For this review, take the finished solid that the model builds, in its own axes (mm). A direction names the side the tool comes from. Coordinates: 2 decimals unless noted, no trailing zeros. Write each loop counter-clockwise with the first axis right and the second up, starting at its lowest first coordinate (ties: lowest second). Pieces come first, ordered by that corner, then holes. Notation, with made-up numbers: M 50,-37 L 76,-37 A17 ccw 76,-33 Z; hole C -33.75,57.25 d5. An arc over 180 degrees is marked long. Return JSON: item names as keys, results as strings.
```python
from build123d import *

# Parameters (mm, degrees)
SKETCH1_R           = 29
BOSS_EXTRUDE1_DEPTH = 5
SKETCH4_R           = 0.9
BOSS_EXTRUDE2_DEPTH = 2.5
SKETCH7_R           = 5
CUT_EXTRUDE4_DEPTH  = 5
SKETCH11_R          = 1
CUT_EXTRUDE6_DEPTH  = 5
SKETCH12_R          = 29
CUT_EXTRUDE7_DEPTH  = 1
SKETCH13_W          = 10
SKETCH13_H          = 10
CUT_EXTRUDE8_DEPTH  = 10
SKETCH14_R          = 29
CUT_EXTRUDE9_DEPTH  = 2.5


with BuildPart() as part:
    # Sketch1 → Boss-Extrude1 (new body)
    with BuildSketch(Plane(origin=(0, 0, 0), x_dir=(1, 0, 0), z_dir=(0, 1, 0))):
        with Locations(Location((0, 0, 0), (0, 0, 270))):
            Circle(SKETCH1_R)
    extrude(amount=BOSS_EXTRUDE1_DEPTH)

    # Sketch4 → Boss-Extrude2 (add)
    with BuildSketch(Plane(origin=(0, 5, 0), x_dir=(1, 0, 0), z_dir=(0, 1, 0))):
        with Locations(Location((8, 0, 0), (0, 0, 270))):
            Circle(SKETCH4_R)
        with Locations(Location((-8, 0, 0), (0, 0, 270))):
            Circle(SKETCH4_R)
        with Locations(Location((0, 8, 0), (0, 0, 270))):
            Circle(SKETCH4_R)
        with Locations(Location((0, -8, 0), (0, 0, 270))):
            Circle(SKETCH4_R)
    extrude(amount=BOSS_EXTRUDE2_DEPTH)

    # Sketch7 → Cut-Extrude4 (cut)
    with BuildSketch(Plane(origin=(0, 5, 0), x_dir=(1, 0, 0), z_dir=(0, 1, 0))):
        with Locations(Location((0, 0, 0), (0, 0, 270))):
            Circle(SKETCH7_R)
    extrude(amount=-CUT_EXTRUDE4_DEPTH, mode=Mode.SUBTRACT)

    # Sketch11 → Cut-Extrude6 (cut)
    with BuildSketch(Plane(origin=(0, 5, 0), x_dir=(1, 0, 0), z_dir=(0, 1, 0))):
        with Locations(Location((-26, 0, 0), (0, 0, 270))):
            Circle(SKETCH11_R)
        with Locations(Location((0, -26, 0), (0, 0, 270))):
            Circle(SKETCH11_R)
        with Locations(Location((26, 0, 0), (0, 0, 270))):
            Circle(SKETCH11_R)
    extrude(amount=-CUT_EXTRUDE6_DEPTH, mode=Mode.SUBTRACT)

    # Sketch12 → Cut-Extrude7 (cut)
    with BuildSketch(Plane(origin=(0, 0, 0), x_dir=(-1, 0, 0), z_dir=(0, -1, 0))):
        with Locations(Location((0, 0, 0), (0, 0, 90))):
            Circle(SKETCH12_R)
    extrude(amount=-CUT_EXTRUDE7_DEPTH, mode=Mode.SUBTRACT)

    # Sketch13 → Cut-Extrude8 (cut)
    with BuildSketch(Plane(origin=(0, 5, 0), x_dir=(1, 0, 0), z_dir=(0, 1, 0))):
        with Locations((0, 24)):
            Rectangle(SKETCH13_W, SKETCH13_H)
    extrude(amount=-CUT_EXTRUDE8_DEPTH, mode=Mode.SUBTRACT)

    # Sketch14 → Cut-Extrude9 (cut)
    with BuildSketch(Plane(origin=(0, 1, 0), x_dir=(-1, 0, 0), z_dir=(0, -1, 0))):
        Circle(SKETCH14_R)
    extrude(amount=-CUT_EXTRUDE9_DEPTH, mode=Mode.SUBTRACT)


solid = part.part
```
1. We need section C-C (y = 5.7). State the section outline as (x, z) points.
Checks:
{"outline": "C -8,0 d1.8; C 0,-8 d1.8; C 0,8 d1.8; C 8,0 d1.8"}
2. We need section A-A (z = 0). State the section outline as (x, y) points, plus the area to 3 significant figures.
Checks:
{"outline": "M -29,3.5 L -27,3.5 L -27,5 L -29,5 Z; M -25,3.5 L -5,3.5 L -5,5 L -7.1,5 L -7.1,7.5 L -8.9,7.5 L -8.9,5 L -25,5 Z; M 5,3.5 L 25,3.5 L 25,5 L 8.9,5 L 8.9,7.5 L 7.1,7.5 L 7.1,5 L 5,5 Z; M 27,3.5 L 29,3.5 L 29,5 L 27,5 Z", "area": "75.0 mm2"}
3. We need section D-D (z = 26). State the section outline as (x, y) points.
Checks:
{"outline": "M -12.85,3.5 L -1,3.5 L -1,5 L -12.85,5 Z; M 1,3.5 L 12.85,3.5 L 12.85,5 L 1,5 Z"}
4. We need section B-B (x = 0). State the section outline as (y, z) points, plus the area to 3 significant figures.
Checks:
{"outline": "M 3.5,-19 L 5,-19 L 5,-8.9 L 7.5,-8.9 L 7.5,-7.1 L 5,-7.1 L 5,-5 L 3.5,-5 Z; M 3.5,5 L 5,5 L 5,7.1 L 7.5,7.1 L 7.5,8.9 L 5,8.9 L 5,25 L 3.5,25 Z; M 3.5,27 L 5,27 L 5,29 L 3.5,29 Z", "area": "63.0 mm2"}
5. Clearance check with flat-ended pins moving along their axes: pin 1 Ø2 at (x, z) = (1.5, 16) entering from +Y; pin 2 Ø0.8 at (x, y) = (-0.5, 4.5) entering from -Z; pin 3 Ø0.8 at (y, z) = (4.5, -23.5) entering from -X. State where each tip first meets the part, or that it passes through.
Checks:
{"pin 1": "y = 5", "pin 2": "z = -19", "pin 3": "x = -17.53"}
6. Wall thickness on L1, parallel to X at y = 3.95, z = 0; L2, parallel to Y at x = 7, z = -17.5; L3, parallel to X at y = 4.7, z = -24: over which ranges is each line inside the solid? List them lowest first. Write a range as from..to.
Checks:
{"L1": "-29..-27, -25..-5, 5..25, 27..29", "L2": "3.5..5", "L3": "-16.28..-5, 5..16.28"}
7. For faces 1 (the face through (0, 7.5, -8)), 2 (the face through (0.27, 6.23, 8.86)), 3 (the face through (5, 4, -24)), list the 3-axis set-ups (+Z, -Z, +X, -X, +Y, -Y) from which the entire face can be reached by the end or side of a thin tool; tool diameter is ignored.
Checks:
{"face 1": "+Z, -Z, +X, -X, +Y", "face 2": "+Y", "face 3": "-Z, +Y, -Y"}
8. Draft analysis for pull direction Z (two halves, no side actions). For faces 4 (the face through (0, 4, 25)), 5 (the face through (8, 7.5, 0)), 6 (the face through (0, 4, -19)), state which applies: +Z half, -Z half, draft (parallel to the pull), parting line (faces both ways), or undercut.
Checks:
{"face 4": "undercut", "face 5": "draft", "face 6": "-Z half"}
